Geometry: final body of the model. Coordinates: model frame, mm. A direction names the side the tool comes from. Round coordinates to 2 decimals unless told otherwise and drop trailing zeros. Loops run counter-clockwise (first coordinate to the right, second up) from the corner with the lowest first, then second, coordinate; pieces in that order, holes last. Notation, with made-up numbers: (34.5, 82) -> (81.5, 82) arc R17 ccw to (81.5, 95) -> close; hole circle Ø9 at (59.25, -32.75). An arc over 180 degrees is marked (long way). Answer in a Markdown table with one row per item.
```python
from build123d import *

# Parameters (mm, degrees)
F1_DEPTH = 63.5
F2_DEPTH = 25.4
F3_DEPTH = 7.9375
F5_R     = 6.35


with BuildPart() as f1:
    # F0 (on Front) → F1 (new body, symmetric)
    with BuildSketch(Plane.XZ):
        Polygon((-41.275, 9.525), (-41.275, -9.525), (41.275, -9.525), (41.275, 9.525), (22.225, 9.525), align=None)
    extrude(amount=F1_DEPTH, both=True)

    # F0 (on Front) → F2 (join, symmetric)
    with BuildSketch(Plane.XZ):
        with BuildLine():
            Line((22.225, 9.525), (41.275, 9.525))
            Line((41.275, 9.525), (41.275, 46.0502))
            ThreePointArc((41.275, 46.0502), (45.92468, 57.27552), (57.15, 61.9252))
            Line((57.15, 61.9252), (60.325, 61.9252))
            Line((60.325, 61.9252), (60.325, 80.9752))
            Line((60.325, 80.9752), (57.15, 80.9752))
            add(Edge.make_bspline(
                [(56.815137, 80.973595), (56.926678, 80.974353), (57.038299, 80.974888), (57.15, 80.9752)],
                knots=[121.334974, 121.334974, 121.334974, 121.334974, 121.624881, 121.624881, 121.624881, 121.624881], degree=3))
            ThreePointArc((56.815137, 80.973595), (32.336186, 70.627227), (22.225, 46.0502))
            Line((22.225, 46.0502), (22.225, 9.525))
        make_face()
        Polygon((85.725, 80.9752), (60.325, 80.9752), (60.325, 61.9252), (71.4375, 61.9252), (85.725, 61.9252), align=None)
    extrude(amount=F2_DEPTH, both=True)

    # F0 (on Front) → F3 (join, symmetric)
    with BuildSketch(Plane.XZ):
        with BuildLine():
            add(Edge.make_bspline(
                [(-41.275, 9.525), (-22.584794, 41.291515), (10.131669, 80.656242), (56.815137, 80.973595)],
                knots=[0, 0, 0, 0, 121.334974, 121.334974, 121.334974, 121.334974], degree=3))
            Line((-41.275, 9.525), (22.225, 9.525))
            Line((22.225, 9.525), (22.225, 46.0502))
            ThreePointArc((22.225, 46.0502), (32.336186, 70.627227), (56.815137, 80.973595))
        make_face()
    extrude(amount=F3_DEPTH, both=True)

    # F0 (on Front) → F4 (revolve)
    with BuildSketch(Plane.XZ):
        Polygon((85.725, 85.725), (85.725, 80.9752), (85.725, 61.9252), (85.725, 57.15), (111.125, 57.15), (111.125, 85.725), align=None)
    revolve(axis=Axis((85.725, 0, 71.4375), (0, 0, 1)))

    # F5
    f5_edges = [f1.edges().sort_by_distance(p)[0] for p in [
        (-41.275, -63.5, 0),
        (41.275, -63.5, 0),
        (41.275, 63.5, 0),
        (-41.275, 63.5, 0),
    ]]
    fillet(f5_edges, radius=F5_R)


solid = f1.part
```
Item 1: First-contact query: P1, Ø5, axis at x = -9, y = 7, coming from the +Z side; P2, Ø21.5, axis at x = 27, z = 51.5, coming from the -Y side; P3, Ø1, axis at x = 54, y = -25, coming from the -Z side; P4, Ø1.5, axis at y = -26.5, z = 45, coming from the -X side. Flat tips, straight axial feed; report the tip coordinate or a pass-through.
Ans:
| item | result |
|---|---|
| P1 | z = 53.72 |
| P2 | y = -25.4 |
| P3 | z = 61.5 |
| P4 | through |
Item 2: Section query A-A, the plane z = 5.5. Output: boundary loops of the cut face in (x, y) (3 decimals).
Ans:
| item | result |
|---|---|
| outline | (-41.275, -57.15) arc R6.35 ccw to (-34.925, -63.5) -> (34.925, -63.5) arc R6.35 ccw to (41.275, -57.15) -> (41.275, 57.15) arc R6.35 ccw to (34.925, 63.5) -> (-34.925, 63.5) arc R6.35 ccw to (-41.275, 57.15) -> close |
Item 3: Ray query, L1, parallel to Z at x = 64.5, y = -17; L2, parallel to Y at x = 27, z = 25; L3, parallel to Z at x = -21, y = 44 (3 decimals). Return the intervals inside material, ascending.
Ans:
| item | result |
|---|---|
| L1 | 61.93 to 80.98 |
| L2 | -25.4 to 25.4 |
| L3 | -9.525 to 9.525 |
Item 4: Set-up query: faces 4 (the flat face through (60, 2, 61.925)), 5 (the flat face through (39, -25.4, 54)), 6 (the flat face through (8, -7.938, 38)), 7 (the flat face through (86, 0, 57.15)), 8 (the flat face through (8, 7.938, 38)). Return all of +Z, -Z, +X, -X, +Y, -Y with unobstructed straight access to the full face (end or side cutting, diameter ignored); none if empty.
Ans:
| item | result |
|---|---|
| face 4 | -Z |
| face 5 | +Z, +X, -X, -Y |
| face 6 | +Z, -X, -Y |
| face 7 | -Z, +X, +Y, -Y |
| face 8 | +Z, -X, +Y |
Item 5: Mould query, pull axis Z, two halves, no side actions, for faces 1 (the cylindrical face through (32.61, 16.55, 70.9)), 2 (the flat face through (-1, -1, -9.525)), 3 (the flat face through (39, 25.4, 54)). Classes: released by +Z, released by -Z, zero draft, split by the parting line, or undercut.
Ans:
| item | result |
|---|---|
| face 1 | released by +Z |
| face 2 | released by -Z |
| face 3 | zero draft |
